Geometry check sheet. Reference: the model listing, model coordinates, mm. A direction names the side the tool comes from. Coordinates: 2 decimals unless noted, no trailing zeros. Write each loop counter-clockwise with the first axis right and the second up, starting at its lowest first coordinate (ties: lowest second). Pieces come first, ordered by that corner, then holes. Notation, with made-up numbers: M 14,65.25 L 21,65.25 A18 ccw 21,84.25 Z; hole C -19,-4 d1. An arc over 180 degrees is marked long. Put each result on its own line as item: value. Start each with the question number.
1) Set-up check for faces 1 (the flat face through (-3, -2.25, 0)), 2 (the conical face through (0.51, 0.83, -3.86)), 3 (the flat face through (3, 2.25, 0)): record each of +Z, -Z, +X, -X, +Y, -Y from which the full face is reachable in a straight line by a thin tool's end or side.
2) Mould release check, pull along Z, two halves, no side actions. Record for faces 4 (the flat face through (-3, 2.25, 0)), 5 (the conical face through (0.51, -0.83, -3.86)), 6 (the flat face through (0.1, 2.75, 2.5)): released by +Z, released by -Z, zero draft, split by the parting line, or undercut.
3) Cross-section at D-D on y = 0.5. Record the cut outline in (x, z).
4) Cross-section at C-C on y = -1.5. Record the cut outline in (x, z).
5) Gauge pin test, flat ends, axial feed: pin 1 (2 mm diameter, centred on y = -2, z = -2.5, fed in from +X); pin 2 (1.7 mm diameter, centred on x = -2, z = 0, fed in from -Y); pin 3 (2 mm diameter, centred on x = -2.5, y = 1, fed in from -Z). Record the tip position at first contact, or that the pin passes through.
6) Scan lines: line 1 along Z through (x, y) = (0, -0.45); line 2 along X through (y, z) = (-0.1, -0.25); line 3 along Y through (x, z) = (-2, -4). Record each from-to range of solid material in increasing order.
7) Cross-section at A-A on x = 0. Record the cut outline in (y, z).
from build123d import *

# Parameters (mm, degrees)
CUT_EXTRUDE_1_DEPTH = 0.5
SKETCH_3_R          = 2
CUT_EXTRUDE_2_DEPTH = 11.111874208
FILLET_1_R          = 0.2


with BuildPart() as part:
    # 草图1 → 旋转1 (revolve)
    with BuildSketch(Plane.XY, mode=Mode.PRIVATE) as revolve_1_sk:
        Polygon((0, 0), (3.75, 0), (3.75, 0.75), (6, 2), (6, 2.75), (0, 2.75), align=None)
    revolve_1 = revolve(revolve_1_sk.sketch.rotate(Axis((0, 2.75, 0), (0, -1, 0)), 180), axis=Axis((0, 2.75, 0), (0, -1, 0)))

    # 镜向1: 旋转1 across plane
    add(revolve_1.mirror(Plane.ZX))

    # 草图2 → 切除-拉伸1 (cut)
    with BuildSketch(Plane(origin=(0, 2.75, 0), x_dir=(1, 0, 0), z_dir=(0, 1, 0))):
        with BuildLine():
            Line((3.16227766, 1.5), (-3.16227766, 1.5))
            ThreePointArc((-3.16227766, 1.5), (-3.5, 0), (-3.16227766, -1.5))
            Line((-3.16227766, -1.5), (3.16227766, -1.5))
            ThreePointArc((3.16227766, -1.5), (3.5, 0), (3.16227766, 1.5))
        make_face()
    cut_extrude_1 = extrude(amount=-CUT_EXTRUDE_1_DEPTH, mode=Mode.SUBTRACT)

    # 镜向2: 切除-拉伸1 across plane
    add(cut_extrude_1.mirror(Plane.ZX), mode=Mode.SUBTRACT)

    # 草图3 → 切除-拉伸2 (cut, through all)
    with BuildSketch(Plane(origin=(0, 2.75, 0), x_dir=(1, 0, 0), z_dir=(0, 1, 0))):
        with Locations(Location((0, 0, 0), (0, 0, 228.590377891))):
            Circle(SKETCH_3_R)
    extrude(amount=-CUT_EXTRUDE_2_DEPTH, mode=Mode.SUBTRACT)

    # 圆角1
    fillet_1_edges = [part.edges().sort_by_distance(p)[0] for p in [
        (6, -2.75, 0),
        (3.5, 2.75, 0),
        (2.242576658, 2.75, -1.5),
        (-3.5, 2.75, 0),
        (-2.242576658, 2.75, 1.5),
        (3.5, -2.75, 0),
        (2.242576658, -2.75, -1.5),
        (-3.5, -2.75, 0),
        (-2.242576658, -2.75, 1.5),
        (2.242576658, -2.75, 1.5),
        (-2.242576658, -2.75, -1.5),
        (6, 2.75, 0),
        (-2.242576658, 2.75, -1.5),
        (2.242576658, 2.75, 1.5),
        (0, 2.75, 2),
        (0, 2.75, -2),
        (0, -2.75, 2),
        (0, -2.75, -2),
    ]]
    fillet(fillet_1_edges, radius=FILLET_1_R)


solid = part.part
Answer key:
1. face 1: -Y
1. face 2: none
1. face 3: +Y
2. face 4: undercut
2. face 5: split by the parting line
2. face 6: zero draft
3. outline: C 0,0 d7.5; hole C 0,0 d4
4. outline: C 0,0 d10.2; hole C 0,0 d4
5. pin 1: stops at x = 5.81
5. pin 2: stops at y = -2.25
5. pin 3: stops at z = -5.5
6. line 1: z = -3.75 to -2, 2 to 3.75
6. line 2: x = -3.74 to -1.98, 1.98 to 3.74
6. line 3: y = -2.75 to -1.15, 1.15 to 2.75
7. outline: M -2.75,-5.8 A0.2 ccw -2.55,-6 L -2,-6 L -0.75,-3.75 L 0.75,-3.75 L 2,-6 L 2.55,-6 A0.2 ccw 2.75,-5.8 L 2.75,-2.2 A0.2 ccw 2.55,-2 L -2.55,-2 A0.2 ccw -2.75,-2.2 Z; M -2.75,2.2 A0.2 ccw -2.55,2 L 2.55,2 A0.2 ccw 2.75,2.2 L 2.75,5.8 A0.2 ccw 2.55,6 L 2,6 L 0.75,3.75 L -0.75,3.75 L -2,6 L -2.55,6 A0.2 ccw -2.75,5.8 Z
